from build123d import *

# Parameters (mm, degrees)
SKETCH1_R                 = 7.5
SKETCH1_R_2               = 2.5
BOSS_EXTRUDE1_DEPTH       = 25
CHAMFER1_SIZE             = 0.5
F_8_32_TAPPED_HOLE1_D     = 3.4544
F_8_32_TAPPED_HOLE1_DEPTH = 18
F_8_32_TAPPED_HOLE1_TIP   = 1.037806461


with BuildPart() as part:
    # Sketch1 → Boss-Extrude1 (new body)
    with BuildSketch(Plane(origin=(0, 0, 0), x_dir=(1, 0, 0), z_dir=(0, 1, 0))):
        Circle(SKETCH1_R)
        Circle(SKETCH1_R_2, mode=Mode.SUBTRACT)
    extrude(amount=BOSS_EXTRUDE1_DEPTH)

    # Chamfer1
    chamfer1_edges = [part.edges().sort_by_distance(p)[0] for p in [
        (-7.5, 0, 0),
        (-7.5, 25, 0),
        (-2.5, 0, 0),
        (-2.5, 25, 0),
    ]]
    chamfer(chamfer1_edges, length=CHAMFER1_SIZE)

    # #8-32 Tapped Hole1
    with Locations(Plane.XY.offset(19.05)):
        with Locations((0, 18), (0, 7)):
            Hole(F_8_32_TAPPED_HOLE1_D / 2, depth=F_8_32_TAPPED_HOLE1_DEPTH)
            with Locations((0, 0, -(F_8_32_TAPPED_HOLE1_DEPTH + F_8_32_TAPPED_HOLE1_TIP / 2))):  # 118° drill point
                Cone(0, F_8_32_TAPPED_HOLE1_D / 2, F_8_32_TAPPED_HOLE1_TIP, mode=Mode.SUBTRACT)


solid = part.part
Build history of the part. All positions in model axes, mm. A direction names the side the tool comes from. Give positions to 0.01 mm unless a question says otherwise; leave off trailing zeros. Order: outer loops, then holes, each group sorted by start corner. A loop starts at its lowest first (then second) coordinate and runs counter-clockwise, first axis right, second up. Notation, with made-up numbers: M 83,31.5 L 140,31.5 A18 cw 140,55.5 Z; hole C -33.75,43.25 d9. An arc over 180 degrees is marked long. Use one line per item in the form item = value.
1) Saw through at A-A (x = 0). Give the cut face in (y, z), plus the area to 3 significant figures.
Calculated:
outline = M 0,-7 L 0.5,-7.5 L 24.5,-7.5 L 25,-7 L 25,-3 L 24.5,-2.5 L 0.5,-2.5 L 0,-3 Z; M 0,3 L 0.5,2.5 L 5.27,2.5 L 5.27,7.5 L 0.5,7.5 L 0,7 Z; M 8.73,2.5 L 16.27,2.5 L 16.27,7.5 L 8.73,7.5 Z; M 19.73,2.5 L 24.5,2.5 L 25,3 L 25,7 L 24.5,7.5 L 19.73,7.5 Z
area = 214 mm2
2) Tool access for faces 4 (the face through (-1.647, 18.519, 4.617)), 5 (the face through (1, 25, 3)): list every direction of +Z, -Z, +X, -X, +Y, -Y with a clear straight run to the whole face (end or side of a thin tool).
Calculated:
face_4 = +Z
face_5 = +Z, -Z, +X, -X, +Y
3) Probe probe 1 along Y at (x, z) = (0, 5.45); probe 2 along Y at (x, z) = (-0.5, 2.5); probe 3 along X at (y, z) = (12, 0). List the from-to ranges inside material, lowest first.
Calculated:
probe_1 = 0 to 5.27, 8.73 to 16.27, 19.73 to 25
probe_2 = 0.45 to 5.35, 8.65 to 16.35, 19.65 to 24.55
probe_3 = -7.5 to -2.5, 2.5 to 7.5
4) Saw through at D-D (y = 6.25). Give the cut face in (x, z), plus the area to 3 significant figures.
Calculated:
outline = M -1.56,1.96 L -1.56,7.34 A7.5 ccw long 1.56,7.34 L 1.56,1.96 A2.5 cw long Z
area = 141 mm2
5) Two-plate mould, pull along Z, no slides. Class faces 1 (the face through (1, 0, 3)), 2 (the face through (-0.976, 12.332, -7.436)), 3 (the face through (-0.33, 12.33, -2.48)): released by +Z, released by -Z, zero draft, split by the parting line, or undercut.
Calculated:
face_1 = zero draft
face_2 = split by the parting line
face_3 = undercut
6) Saw through at B-B (z = 0). Give the cut face in (x, y), plus the area to 3 significant figures.
Calculated:
outline = M -7.5,0.5 L -7,0 L -3,0 L -2.5,0.5 L -2.5,24.5 L -3,25 L -7,25 L -7.5,24.5 Z; M 2.5,0.5 L 3,0 L 7,0 L 7.5,0.5 L 7.5,24.5 L 7,25 L 3,25 L 2.5,24.5 Z
area = 249 mm2
7) Saw through at C-C (y = 11.75). Give the cut face in (x, z), plus the area to 3 significant figures.
Calculated:
outline = C 0,0 d15; hole C 0,0 d5
area = 157 mm2
8) Drop flat-ended pins along their axis: pin 1 (4 mm diameter, centred on x = -3.5, y = 3.5, fed in from +Z); pin 2 (1 mm diameter, centred on y = 17.5, z = 1.5, fed in from -X); pin 3 (3 mm diameter, centred on x = 0, y = 7, fed in from +Z). Give the stop position or say it passes through.
Calculated:
pin_1 = 7.35
pin_2 = -7.43
pin_3 = -2
